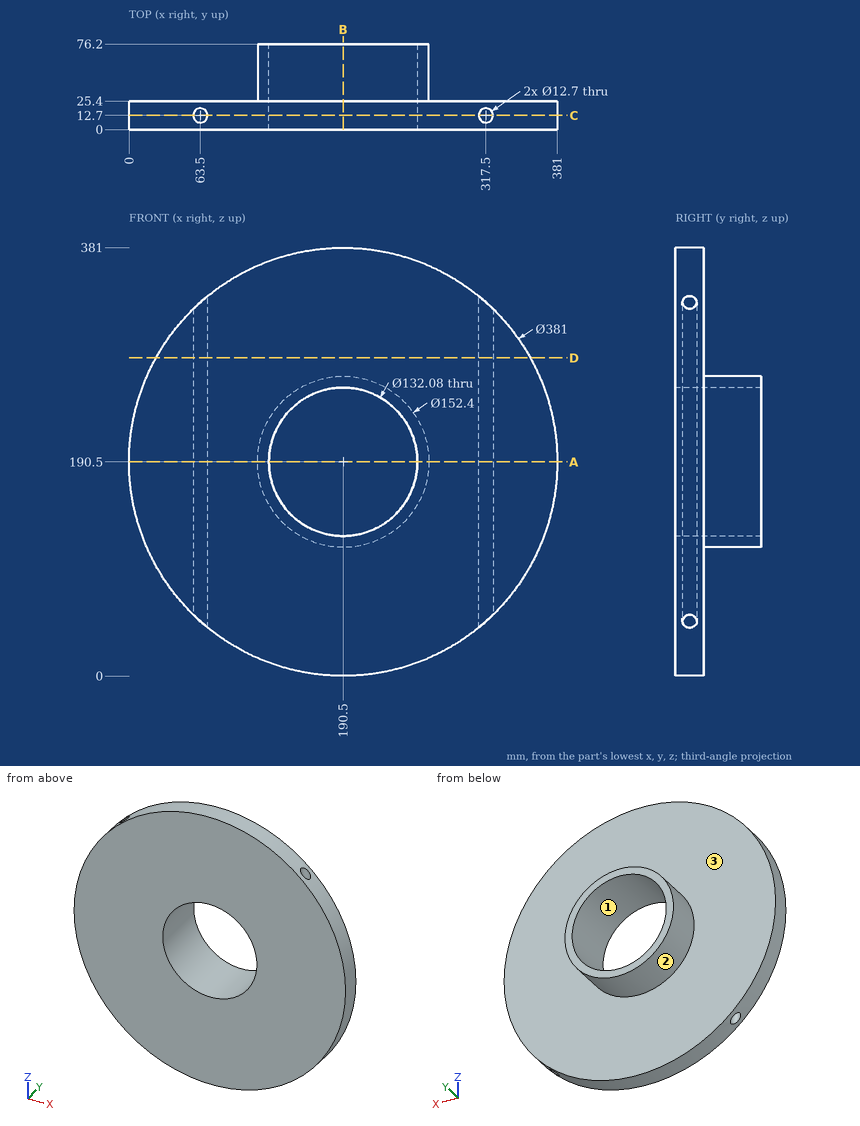
Print and shaded views of the part. All mm, measured from the part's lowest x, y and z. Coordinates: 2 decimals unless noted, no trailing zeros. Write each loop counter-clockwise with the first axis right and the second up, starting at its lowest first coordinate (ties: lowest second). Pieces come first, ordered by that corner, then holes. Notation, with made-up numbers: (89.25, 56.25) - (136.25, 56.25) arc R31 ccw to (136.25, 84.25) - close; hole circle Ø4 at (87.5, 34). An arc over 180 degrees is marked (long way). One line per question, with ' | ' between items. Start each with the question number.
Q1. Pin check, flat tips, straight feed: pin 1 (10 mm diameter, centred on y = 52.5, z = 259, fed in from +X); pin 2 (2 mm diameter, centred on x = 40.5, z = 188.5, fed in from +Y); pin 3 (4 mm diameter, centred on x = 158.5, y = 56.5, fed in from -Z). Stop position of each tip, or through.
Q2. Cut at B-B, the plane x = 190.5. List the corners of the cut face in (y, z), then the cut area to 3 significant figures.
Q3. Cut at D-D, the plane z = 283. List the corners of the cut face in (x, y).
Q4. Cut at C-C, the plane y = 12.7. List the corners of the cut face in (x, z).
Q5. Cut at A-A, the plane z = 190.5. List the corners of the cut face in (x, y), then the cut area to 3 significant figures.
Q6. Drill centre lines: line 1 (Y direction, x = 63, z = 138); line 2 (X direction, y = 44.5, z = 193); line 3 (X direction, y = 7, z = 265). Where is each one in solid material? Low to high. Write a range as [from, to].
Q7. Pull direction X, two halves, no side cores. Call the marked faces 1, 2 and 3: pulls with the +X half, pulls with the -X half, needs draft (parallel to the pull), parting line crosses it, or undercut.
Answer below:
1) pin 1: x = 232.62 | pin 2: y = 25.4 | pin 3: z = 120.45
2) outline: (0, 0) - (25.4, 0) - (25.4, 114.3) - (76.2, 114.3) - (76.2, 124.46) - (0, 124.46) - close; (0, 256.54) - (76.2, 256.54) - (76.2, 266.7) - (25.4, 266.7) - (25.4, 381) - (0, 381) - close | area: 7,350 mm^2
3) outline: (23.96, 0) - (357.04, 0) - (357.04, 25.4) - (23.96, 25.4) - close; hole circle Ø12.7 at (63.5, 12.7); hole circle Ø12.7 at (317.5, 12.7)
4) outline: (57.15, 54.46) - (57.15, 326.54) arc R190.5 ccw to start; (69.85, 43.08) arc R190.5 ccw to (311.15, 43.08) - (311.15, 337.92) arc R190.5 ccw to (69.85, 337.92) - close; (323.85, 54.46) arc R190.5 ccw to (323.85, 326.54) - close; hole circle Ø132.08 at (190.5, 190.5)
5) outline: (0, 0) - (124.46, 0) - (124.46, 76.2) - (114.3, 76.2) - (114.3, 25.4) - (0, 25.4) - close; (256.54, 0) - (381, 0) - (381, 25.4) - (266.7, 25.4) - (266.7, 76.2) - (256.54, 76.2) - close; hole circle Ø12.7 at (63.5, 12.7); hole circle Ø12.7 at (317.5, 12.7) | area: 7,100 mm^2
6) line 1: [0, 6.37], [19.03, 25.4] | line 2: [114.34, 124.51], [256.49, 266.66] | line 3: [15.17, 60.7], [66.3, 314.7], [320.3, 365.83]
7) face 1: undercut | face 2: parting line crosses it | face 3: needs draft
